```python
from build123d import *

# Parameters (mm, degrees)
CROQUIS_BASE_W             = 125
CROQUIS_BASE_H             = 75
CAJA_BAJA_DEPTH            = 50
CROQUIS_AGUJEROS_MONTAJE_R = 4
AGUJERO_INSERTO_M6_DEPTH   = 14


with BuildPart() as part:
    # Croquis_base → Caja_baja (new body)
    with BuildSketch(Plane(origin=(0, 0, 0), x_dir=(1, 0, 0), z_dir=(0, 1, 0))):
        Rectangle(CROQUIS_BASE_W, CROQUIS_BASE_H)
    extrude(amount=CAJA_BAJA_DEPTH)

    # Croquis_agujeros_montaje → Agujero_inserto_M6 (cut)
    with BuildSketch(Plane(origin=(0, 0, 0), x_dir=(1, 0, 0), z_dir=(0, 1, 0))):
        with Locations(Location((-50, 0, 0), (0, 0, 270))):
            Circle(CROQUIS_AGUJEROS_MONTAJE_R)
        with Locations(Location((50, 0, 0), (0, 0, 270))):
            Circle(CROQUIS_AGUJEROS_MONTAJE_R)
    extrude(amount=AGUJERO_INSERTO_M6_DEPTH, mode=Mode.SUBTRACT)


solid = part.part
```
Verification items for the finished model (mm, model axes). A direction names the side the tool comes from. Give positions to 0.01 mm unless a question says otherwise; leave off trailing zeros. Write each loop counter-clockwise with the first axis right and the second up, starting at its lowest first coordinate (ties: lowest second). Pieces come first, ordered by that corner, then holes. Notation, with made-up numbers: (55, 71) - (112, 71) arc R8 cw to (112, 80) - close; hole circle Ø9 at (19, 85.5). An arc over 180 degrees is marked (long way). Put each result on its own line as item: value.
Q1. Scan lines: probe 1 along X at (y, z) = (5.75, 0); probe 2 along Y at (x, z) = (50.5, -0.5). Record each from-to range of solid material in increasing order. Write a range as from..to.
Result:
probe 1: -62.5..-54, -46..46, 54..62.5
probe 2: 14..50
Q2. Section check A-A on x = 50. Record the cut outline in (y, z), and give its area (3 significant figures).
Result:
outline: (0, -37.5) - (50, -37.5) - (50, 37.5) - (0, 37.5) - (0, 4) - (14, 4) - (14, -4) - (0, -4) - close
area: 3,640 mm2
Q3. Set-up check for faces 4 (the face through (-1, 25, 37.5)), 5 (the face through (-52.4, 6.9, -3.2)): record each of +Z, -Z, +X, -X, +Y, -Y from which the full face is reachable in a straight line by a thin tool's end or side.
Result:
face 4: +Z, +X, -X, +Y, -Y
face 5: -Y
Q4. Mould release check, pull along Z, two halves, no side actions. Record for faces 1 (the face through (-1, 0, -1)), 2 (the face through (-50, 14, 0)), 3 (the face through (-1, 25, -37.5)): released by +Z, released by -Z, zero draft, split by the parting line, or undercut.
Result:
face 1: zero draft
face 2: undercut
face 3: released by -Z
Q5. Section check B-B on z = 0. Record the cut outline in (x, y), and give its area (3 significant figures).
Result:
outline: (-62.5, 0) - (-54, 0) - (-54, 14) - (-46, 14) - (-46, 0) - (46, 0) - (46, 14) - (54, 14) - (54, 0) - (62.5, 0) - (62.5, 50) - (-62.5, 50) - close
area: 6,030 mm2
Q6. Depth check by flat-ended pin: P1, Ø2.5, axis at x = 49.5, z = -0.5, coming from the -Y side; P2, Ø9, axis at x = -50, z = 0, coming from the -Y side. Enter the tip coordinate at first touch or a pass-through.
Result:
P1: y = 14
P2: y = 0
